Autodesk Inventor part; units mm, degrees
ref_plane "Work Plane1" through (29, 0, 0) normal (0, -1, 0) x (1, 0, 0)
ref_plane "YZ Plane" through (0, 0, 0) normal (1, 0, 0) x (0, 1, 0)
ref_plane "XZ Plane" through (0, 0, 0) normal (0, 1, 0) x (-1, 0, 0)
sketch "Sketch1" plane through (0, 0, 0) normal (0, 0, 1) x (1, 0, 0)
  line L0 (-1.2192, 0) -> (15.875, 0)
  line L1 (15.875, 0) -> (15.875, 2.413)
  line L2 (15.875, 2.413) -> (2.6461, 2.413)
  line L3 (2.6461, 2.413) -> (0.0001, 2.413)
  line L4 (0.0001, 2.413) -> (0, 2.413)
  line L5 (0, 2.413) -> (0, 3.9624)
  line L6 (0, 3.9624) -> (-4.826, 3.9624)
  line L7 (-4.826, 3.9624) -> (-4.826, 2.2877)
  line L8 (-4.826, 2.2877) -> (-2.54, 2.2877)
  line L9 (-2.54, 2.2877) -> (-1.2192, 0)
  line L10 (-8.9662, 0) -> (20.0152, 0)
  line L11 (0, -0.7925) -> (0, 4.7549)
  line L12 (2.6461, 2.413) -> (0, 2.413) construction
  dimension "d1" = 13.2289
  dimension "d2" = 2.646
  dimension "d3" = 4.826
  dimension "d4" = 2.286
  dimension "d5" = 60
  dimension "d6" = 4.826
  dimension "d7" = 4.826
  dimension "d8" = 4.5754
  dimension "d9" = 7.9248
  dimension "d26" = 15.875
revolve "Body" add sketch "Sketch1" angle 360 about axis through (-1.2192, 0, 0) along (1, 0, 0)
sketch "Sketch2" plane through (-4.826, 0, 0) normal (-1, 0, 0) x (0, 0, 1)
  circle A0 centre (0, 0) radius 2.2877
  line L0 (0, -5.5474) -> (0, 5.5474)
  line L1 (-5.5474, 0) -> (5.5474, 0)
  line L2 (2.2877, 0) -> (1.1438, -1.9812)
  line L3 (1.1438, -1.9812) -> (-1.1438, -1.9812)
  line L4 (-1.1438, -1.9812) -> (-2.2877, 0)
  line L5 (-2.2877, 0) -> (-1.1438, 1.9812)
  line L6 (-1.1438, 1.9812) -> (1.1438, 1.9812)
  line L7 (1.1438, 1.9812) -> (2.2877, 0)
extrude "Slot" add sketch "Sketch2" against normal up to next contours L7 A0 | A0 L2 | L6 L0 A0 | A0 L0 L3 | L0 L6 A0 | A0 L3 L0 | L4 A0 | A0 L5
fillet "Fillet1" radius 0.4572 1 edges at (-4.826, -3.9624, 0)
thread "Thread"
chamfer "Chamfer1" distance 0.6299 distance2 0.6299 1 edges at (15.875, -2.413, 0) measured on face at (15.875, -1.2173, -0.6389)
ref_plane "Work Plane1" through (29, 0, 0) normal (0, -1, 0) x (1, 0, 0)
fillet "Fillet2" radius 0.1524 1 edges at (0.0001, -2.413, 0)
equation "\"d30\" = R"
equation "\"d17\" = RR"
equation "\"d13\" = GEL"
equation "\"d15\" = -0.5 * SPD + 0.5 * GD"
equation "\"d16\" = GUL"
equation "\"d1\" = GEL"
equation "\"d3\" = KOH"
equation "\"d4\" = INTI"
equation "\"d6\" = GD"
equation "\"d7\" = BDM"
equation "\"d8\" = 1.1547 * SW"
equation "\"d9\" = KOD"
equation "\"d26\" = NLG"
equation "\"GD\" = 4.826"
equation "\"NLG\" = 15.875"
equation "\"GEL\" = 13.22888"
equation "\"KOD\" = 7.9248"
equation "\"KOH\" = 4.826"
equation "\"INTI\" = 2.286"
equation "\"GAL\" = 2.64592"
equation "\"GUL\" = 0.62992"
equation "\"BDM\" = 4.826"
equation "\"SW\" = 3.9624"
equation "\"RR\" = 0.4572"
equation "\"SPD\" = 3.56616"
equation "\"R\" = 0.1524"
equation "\"PHH\" = 0.127"
equation "\"GD1\" = SPD"
equation "\"THREADDIA\" = 4.826"
equation "\"FAWI\" = 45deg"
equation "\"KOH1\" = 4.3434"
equation "\"NND\" = 4.826"
equation "\"TOA\" = 30deg"
equation "\"E0\" = 1.155 * SW"
properties part number "am-1120" material "Steel, Mild"
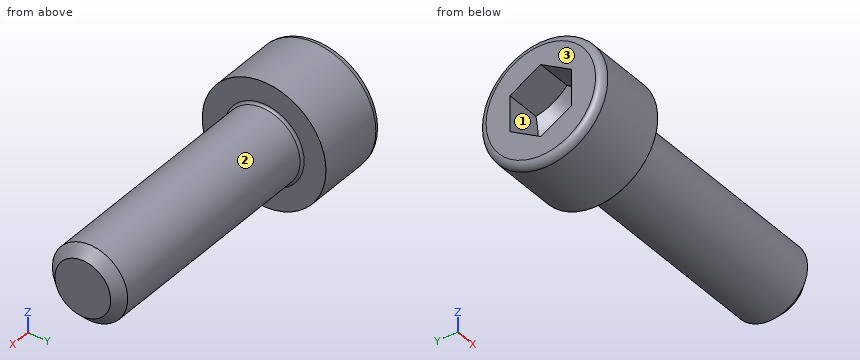
The model under review builds one solid part; all positions refer to its coordinate system, in mm. Face numbers are marked on the shaded views. A direction names the side the tool comes from. Round coordinates to 2 decimals unless told otherwise and drop trailing zeros. Write each loop counter-clockwise with the first axis right and the second up, starting at its lowest first coordinate (ties: lowest second). Pieces come first, ordered by that corner, then holes. Notation, with made-up numbers: M 26,48 L 85,48 A19 cw 85,61 Z; hole C 61,73 d3. An arc over 180 degrees is marked long. Use a Markdown table: item, result. Add a question column.
Q1. Machinability: for the marked faces 1, 2 and 3, which of the approach directions +Z, -Z, +X, -X, +Y, -Y give a long, thin tool a straight path to every point of the face, cutting with its end or side? Answer none if there is none.
Q2. We need section A-A, the plane x = -1.5. State the section outline as (y, z) points.
Q3. To check wall thickness, follow line 1 (X direction, y = -3, z = 0); line 2 (Z direction, x = -1.75, y = -0.25); line 3 (Z direction, x = 5.5, y = -0.75). State the ranges of each line that lie inside material, in increasing order.
Q4. Insertion check: pin 1 (0.7 mm diameter, centred on x = -4, z = 0.5, fed in from -Y); pin 2 (3 mm diameter, centred on x = 13.5, z = -1.5, fed in from +Y); pin 3 (1 mm diameter, centred on y = 0.5, z = 0.5, fed in from -X). Each pin has a flat end and moves straight along its axis. Give the tip position at first contact, or say it passes through.
Q5. We need section B-B, the plane x = 5.5. State the section outline as (y, z) points.
Findings below:
| question | item | result |
|---|---|---|
| 1 | face 1 | -X |
| 1 | face 2 | +X |
| 1 | face 3 | +Z, -Z, -X, +Y, -Y |
| 2 | outline | C 0,0 d7.92; hole C 0,0 d0.97 |
| 3 | line 1 | x = -4.83 to 0 |
| 3 | line 2 | z = -3.95 to -0.88, 0.88 to 3.95 |
| 3 | line 3 | z = -2.29 to 2.29 |
| 4 | pin 1 | stops at y = -3.96 |
| 4 | pin 2 | stops at y = 2.41 |
| 4 | pin 3 | stops at x = -1.92 |
| 5 | outline | C 0,0 d4.83 |
